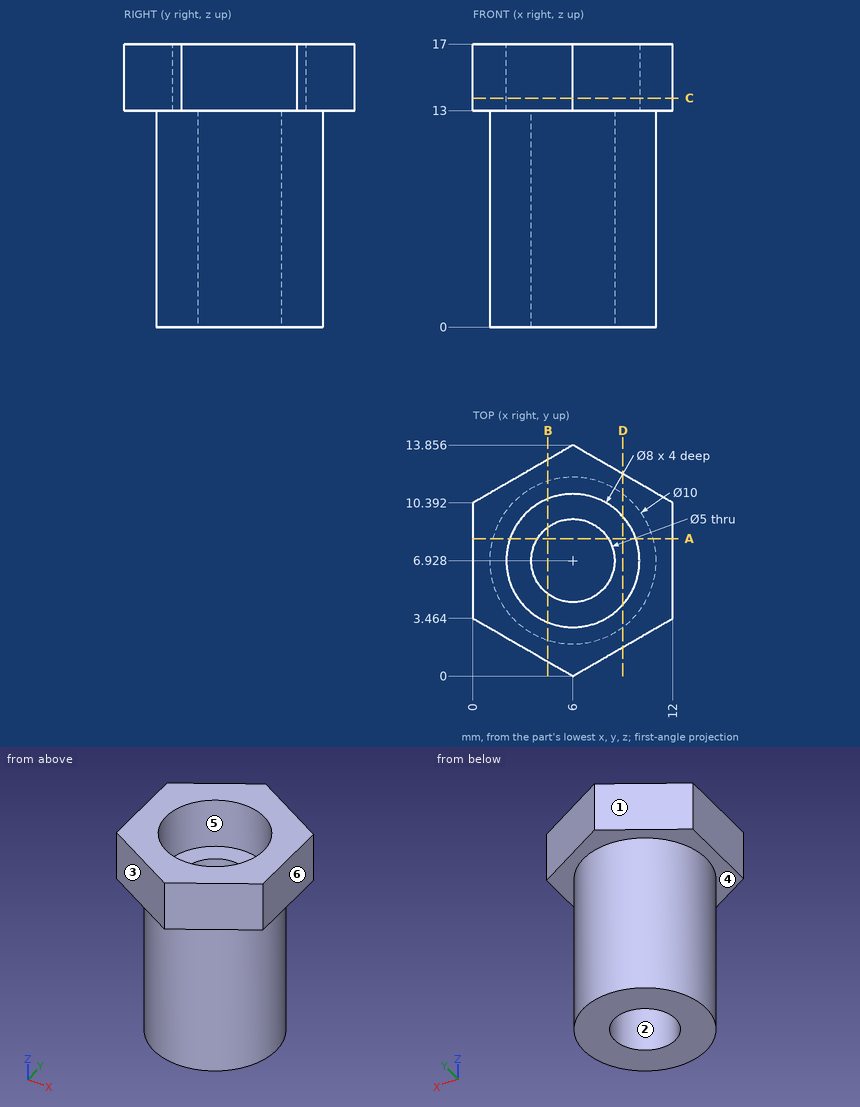
Source: three-view drawing plus pictorial views. Frame: mm from the lowest corner of the part. A direction names the side the tool comes from. Round coordinates to 2 decimals unless told otherwise and drop trailing zeros. Order: outer loops, then holes, each group sorted by start corner. A loop starts at its lowest first (then second) coordinate and runs counter-clockwise, first axis right, second up. Notation, with made-up numbers: (45, -32.5) - (75, -32.5) arc R20 cw to (75, -1.5) - close; hole circle Ø4 at (70, 14). An arc over 180 degrees is marked (long way). Use a Markdown table: item, result.
1. Section C-C on z = 13.75. Return the cut outline in (x, y).
Evaluation:
| item | result |
|---|---|
| outline | (0, 3.46) - (6, 0) - (12, 3.46) - (12, 10.39) - (6, 13.86) - (0, 10.39) - close; hole circle Ø8 at (6, 6.93) |
2. Material intervals for probe 1 along Y at (x, z) = (6, 4); probe 2 along Z at (x, y) = (8.75, 12); probe 3 along Z at (x, y) = (9.25, 8.75), sorted ascending.
Evaluation:
| item | result |
|---|---|
| probe 1 | 1.93 to 4.43, 9.43 to 11.93 |
| probe 2 | 13 to 17 |
| probe 3 | 0 to 13 |
3. Section A-A on y = 8.25. Return the cut outline in (x, z) (1 decimal).
Evaluation:
| item | result |
|---|---|
| outline | (0, 13) - (1.2, 13) - (1.2, 0) - (3.9, 0) - (3.9, 13) - (2.2, 13) - (2.2, 17) - (0, 17) - close; (8.1, 0) - (10.8, 0) - (10.8, 13) - (12, 13) - (12, 17) - (9.8, 17) - (9.8, 13) - (8.1, 13) - close |
4. Mould query, pull axis Y, two halves, no side actions, for the marked faces 1, 2 and 3. Classes: +Y half, -Y half, draft (parallel to the pull), parting line (faces both ways), or undercut.
Evaluation:
| item | result |
|---|---|
| face 1 | +Y half |
| face 2 | undercut |
| face 3 | -Y half |
5. Section B-B on x = 4.5. Return the cut outline in (y, z).
Evaluation:
| item | result |
|---|---|
| outline | (0.87, 13) - (2.16, 13) - (2.16, 0) - (4.93, 0) - (4.93, 13) - (3.22, 13) - (3.22, 17) - (0.87, 17) - close; (8.93, 0) - (11.7, 0) - (11.7, 13) - (12.99, 13) - (12.99, 17) - (10.64, 17) - (10.64, 13) - (8.93, 13) - close |
6. First-contact query: pin 1 (4 mm diameter, centred on x = 5.5, y = 6, fed in from +Z); pin 2 (1.5 mm diameter, centred on x = 6, z = 9, fed in from +Y); pin 3 (1 mm diameter, centred on y = 6, z = 7.5, fed in from +X). Flat tips, straight axial feed; report the tip coordinate or a pass-through.
Evaluation:
| item | result |
|---|---|
| pin 1 | z = 13 |
| pin 2 | y = 11.93 |
| pin 3 | x = 10.98 |
7. Access query for the marked faces 4, 5 and 6. Directions: +Z, -Z, +X, -X, +Y, -Y. A direction counts if a zero-diameter tool reaches every point of the face in a straight line with its end or side. Return the directions, or none.
Evaluation:
| item | result |
|---|---|
| face 4 | -Z |
| face 5 | +Z |
| face 6 | +Z, -Z, +X, +Y, -Y |
8. Section D-D on x = 9. Return the cut outline in (y, z) (1 decimal), then the cut area to 3 significant figures.
Evaluation:
| item | result |
|---|---|
| outline | (1.7, 13) - (2.9, 13) - (2.9, 0) - (10.9, 0) - (10.9, 13) - (12.1, 13) - (12.1, 17) - (9.6, 17) - (9.6, 13) - (4.3, 13) - (4.3, 17) - (1.7, 17) - close |
| area | 124 mm^2 |
